Part model, mm, in its own coordinate system. Round coordinates to 2 decimals unless told otherwise and drop trailing zeros. Loops run counter-clockwise (first coordinate to the right, second up) from the corner with the lowest first, then second, coordinate; pieces in that order, holes last. Notation, with made-up numbers: M 84,8.25 L 106,8.25 A26 ccw 106,34.25 Z; hole C 41,-33.5 d2. An arc over 180 degrees is marked long. Answer as CSV lines item,"result". Start each with the question number.
Item 1: Drop flat-ended pins along their axis: pin 1 Ø2.5 at (y, z) = (6, 24.5) entering from +X; pin 2 Ø10 at (x, z) = (17.5, 20) entering from -Y; pin 3 Ø12 at (x, z) = (3, -9.5) entering from +Y; pin 4 Ø1.5 at (y, z) = (5, 21.5) entering from -X. Give the stop position or say it passes through.
Item 2: Band-saw the part on C-C (x = 5). Give the cut face in (y, z).
Item 3: Wall check: line 1 (Y direction, x = 4.5, z = 16); line 2 (X direction, y = 5, z = 23.5); line 3 (Z direction, x = 2.5, y = 4.25). Give the ranges that are in metal, low to high.
Item 4: Band-saw the part on B-B (z = -2). Give the cut face in (x, y), and give its area (3 significant figures).
Item 5: Band-saw the part on A-A (x = 14). Give the cut face in (y, z).
Autodesk Inventor part; units mm, degrees
ref_plane "YZ Plane" through (0, 0, 0) normal (1, 0, 0) x (0, 1, 0)
ref_plane "XZ Plane" through (0, 0, 0) normal (0, 1, 0) x (-1, 0, 0)
ref_plane "XY Plane" through (0, 0, 0) normal (0, 0, 1) x (1, 0, 0)
sketch "Sketch1" plane through (0, 0, 0) normal (0, 1, 0) x (-1, 0, 0)
  line L0 (-22.5, -28) -> (22.5, -28)
  line L1 (22.5, -28) -> (22.5, 28)
  line L2 (22.5, 28) -> (-22.5, 28)
  line L3 (-22.5, 28) -> (-22.5, -28)
  line L4 (-22.5, -28) -> (22.5, 28) construction
  line L5 (22.5, -28) -> (-22.5, 28) construction
  point P0 (0, 0)
  dimension "d0" = 56
  dimension "d1" = 45
extrude "Extrusion1" add sketch "Sketch1" along normal blind 4
sketch "Sketch2" plane through (0, 4, 0) normal (0, 1, 0) x (1, 0, 0)
  line L0 (-6.25, -28) -> (6.25, -28)
  line L1 (6.25, -28) -> (6.25, -18)
  line L2 (6.25, -18) -> (-6.25, -18)
  line L3 (-6.25, -18) -> (-6.25, -28)
  line L4 (-22.5, -28) -> (22.5, -28)
  point P0 (0, 0)
  point P1 (0, -18)
  dimension "d4" = 12.5
  dimension "d5" = 10
extrude "Extrusion2" add sketch "Sketch2" along normal blind 3
properties part number "BMS"
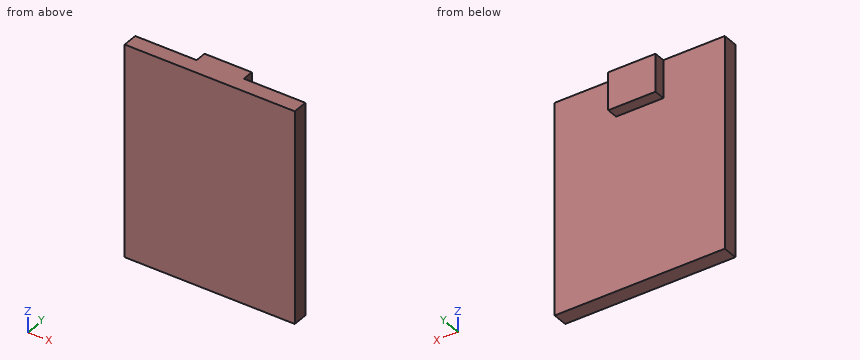
Answer block:
1,pin 1,"stops at x = 6.25"
1,pin 2,"stops at y = 0"
1,pin 3,"stops at y = 4"
1,pin 4,"stops at x = -6.25"
2,outline,"M 0,-28 L 4,-28 L 4,18 L 7,18 L 7,28 L 0,28 Z"
3,line 1,"y = 0 to 4"
3,line 2,"x = -6.25 to 6.25"
3,line 3,"z = 18 to 28"
4,outline,"M -22.5,0 L 22.5,0 L 22.5,4 L -22.5,4 Z"
4,area,"180 mm^2"
5,outline,"M 0,-28 L 4,-28 L 4,28 L 0,28 Z"
